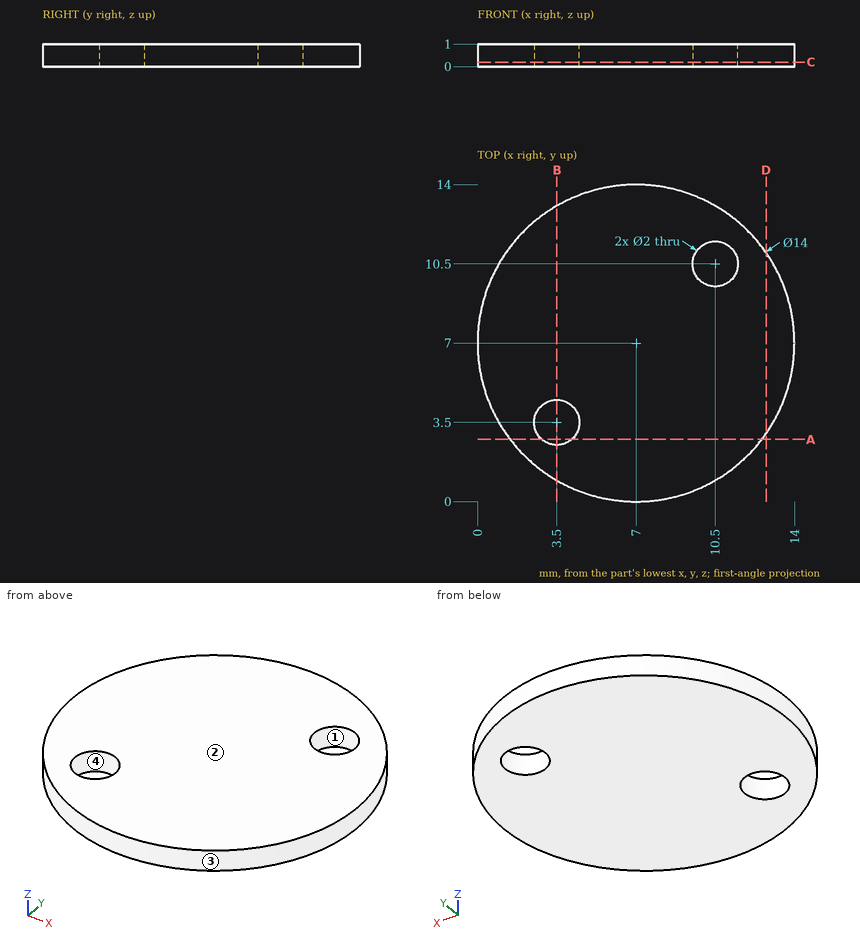
Could you check a few things on this drawing? It's one solid part, dimensions in mm from its lowest x, y, z. Give positions to 0.01 mm unless a question says otherwise; leave off trailing zeros. Loops run counter-clockwise (first coordinate to the right, second up) from the corner with the lowest first, then second, coordinate; pieces in that order, holes last. Notation, with made-up numbers: (-6.75, -28.75) -> (4.25, -28.75) arc R27 cw to (4.25, -3.75) -> close; hole circle Ø5 at (-9, 2.25). An arc over 180 degrees is marked (long way). Use one line per item in the form item = value. Start each with the question number.
1) Please list where these lines run through material, in increasing order: line 1 along X through (y, z) = (2.75, 0.55); line 2 along X through (y, z) = (3.5, 0.25).
2) Imagine slicing it at A-A (y = 2.75). Please give me the cut outline in (x, z), then the cut area to 3 significant figures.
3) Imagine slicing it at B-B (x = 3.5). Please give me the cut outline in (y, z).
4) Imagine slicing it at D-D (x = 12.75). Please give me the cut outline in (y, z).
5) Imagine slicing it at C-C (z = 0.2). Please give me the cut outline in (x, y), then the cut area to 3 significant figures.
6) Thinking about a two-plate mould opening in X: for the marked faces 1, 2, 3 and 4, which applies, +X half, -X half, draft (parallel to the pull), parting line (faces both ways), or undercut?
Check values:
q1.line_1 = 1.44 to 2.84, 4.16 to 12.56
q1.line_2 = 0.94 to 2.5, 4.5 to 13.06
q2.outline = (1.44, 0) -> (2.84, 0) -> (2.84, 1) -> (1.44, 1) -> close; (4.16, 0) -> (12.56, 0) -> (12.56, 1) -> (4.16, 1) -> close
q2.area = 9.80 mm^2
q3.outline = (0.94, 0) -> (2.5, 0) -> (2.5, 1) -> (0.94, 1) -> close; (4.5, 0) -> (13.06, 0) -> (13.06, 1) -> (4.5, 1) -> close
q4.outline = (3.01, 0) -> (10.99, 0) -> (10.99, 1) -> (3.01, 1) -> close
q5.outline = circle Ø14 at (7, 7); hole circle Ø2 at (3.5, 3.5); hole circle Ø2 at (10.5, 10.5)
q5.area = 148 mm^2
q6.face_1 = undercut
q6.face_2 = draft
q6.face_3 = parting line
q6.face_4 = undercut
